Geometry: final body of the model. Coordinates: model frame, mm. A direction names the side the tool comes from. Coordinates: 2 decimals unless noted, no trailing zeros. Loops run counter-clockwise (first coordinate to the right, second up) from the corner with the lowest first, then second, coordinate; pieces in that order, holes last. Notation, with made-up numbers: (-40, 12.5) - (-32, 12.5) arc R20 ccw to (-32, 28.5) - close; hole circle Ø8 at (47, 8). An arc over 180 degrees is marked (long way). Put each result on its own line as item: value. Start each with the question number.
1) Contact query for flat-ended pins moving along their axis: pin 1 Ø4 at (x, y) = (7.5, -20.5) entering from +Z; pin 2 Ø6 at (x, y) = (15.5, -20) entering from +Z; pin 3 Ø12 at (y, z) = (-7.5, -14.5) entering from +X. Output: stop coordinate, or through.
2) Draft query along X for faces 1 (the cylindrical face through (0.701, -27.384, 1.765)), 2 (the flat face through (-3, -4.9, 3)), 3 (the cylindrical face through (0, -15, 0)). Return one class per face: +X half, -X half, draft (parallel to the pull), parting line (faces both ways), or undercut.
3) Material intervals for line 1 along Z through (x, y) = (-1.6, -7.75); line 2 along Y through (x, z) = (-0.5, -16); line 3 along Z through (x, y) = (-1.6, -23.5), sorted ascending. Write a range as from..to.
4) Reachability of faces 4 (the flat face through (-2, -6.9, 10)), 5 (the flat face through (-1, -22.9, 10)), 6 (the cylindrical face through (-23.538, -15.012, -6.909)) from +Z, -Z, +X, -X, +Y, -Y: full face, straight path, thin tool, end or side. Return the list, or none.
5) Section D-D on x = 7.5. Output: boundary loops of the cut face in (y, z).
6) Section C-C on y = -2. Output: boundary loops of the cut face in (x, z).
```python
from build123d import *

# Parameters (mm, degrees)
FILLET_1_R = 2


with BuildPart() as part:
    # 草图1 → 旋转1 (revolve)
    with BuildSketch(Plane.XY, mode=Mode.PRIVATE) as revolve_1_sk:
        Polygon((0, 0), (1.3, 0), (1.3, -4.9), (4.4, -4.9), (4.4, -6.9), (21.4, -6.9), (21.4, -22.9), (4.4, -22.9), (4.4, -24.9), (1.3, -24.9), (1.3, -29.8), (0, -29.8), align=None)
    revolve(revolve_1_sk.sketch.rotate(Axis((-1.6, 5.739994567, 0), (0, -1, 0)), 180), axis=Axis((-1.6, 5.739994567, 0), (0, -1, 0)))

    # 圆角1
    fillet_1_edges = [part.edges().sort_by_distance(p)[0] for p in [
        (4.4, -22.9, 0),
        (4.4, -6.9, 0),
    ]]
    fillet(fillet_1_edges, radius=FILLET_1_R - 0.0001)  # a hair under: the kernel refuses the full size


solid = part.part
```
Answer block:
1. pin 1: stops at z = 21.88
1. pin 2: stops at z = 18.17
1. pin 3: stops at x = 19.77
2. face 1: parting line
2. face 2: draft
2. face 3: undercut
3. line 1: z = -23..-1.6, 1.6..23
3. line 2: y = -22.9..-6.9
3. line 3: z = -6.57..-1.6, 1.6..6.57
4. face 4: +Y
4. face 5: -Y
4. face 6: +Y, -Y
5. outline: (-22.9, -21.12) - (-6.9, -21.12) - (-6.9, 21.12) - (-22.9, 21.12) - close
6. outline: circle Ø5.8 at (-1.6, 0); hole circle Ø3.2 at (-1.6, 0)
